Verification items for the finished model (mm, model axes). Coordinates: 2 decimals unless noted, no trailing zeros. Write each loop counter-clockwise with the first axis right and the second up, starting at its lowest first coordinate (ties: lowest second). Pieces come first, ordered by that corner, then holes. Notation, with made-up numbers: (30.5, 0.25) -> (88.5, 0.25) arc R24 ccw to (88.5, 26.25) -> close; hole circle Ø5 at (-11, 85). An arc over 180 degrees is marked (long way). Use CSV: the item, a comma, the result in double quotes.
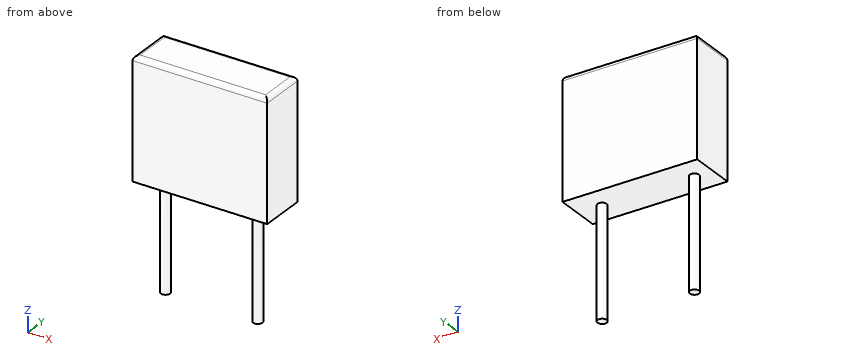
```python
from build123d import *

# Parameters (mm, degrees)
SKETCH_W     = 7.3
SKETCH_H     = 2.5
PAD_DEPTH    = 6.5
FILLET_R     = 0.25
SKETCH001_R  = 0.25
PAD001_DEPTH = 6


with BuildPart() as part:
    # Sketch → Pad (new body)
    with BuildSketch(Plane.XY):
        with Locations((0.178171, 0)):
            Rectangle(SKETCH_W, SKETCH_H)
    extrude(amount=PAD_DEPTH)

    # Fillet
    fillet_edges = [part.edges().sort_by_distance(p)[0] for p in [
        (0.178171, -1.25, 6.5),
        (0.178171, 1.25, 6.5),
        (3.828171, 0, 6.5),
        (-3.471829, 0, 6.5),
    ]]
    fillet(fillet_edges, radius=FILLET_R)

    # Sketch001 (on Face4 of Fillet) → Pad001 (join)
    with BuildSketch(Plane(origin=(0, 0, 0), x_dir=(1, 0, 0), z_dir=(0, 0, -1))):
        with Locations((2.5, 0)):
            Circle(SKETCH001_R)
        with Locations((-2.5, 0)):
            Circle(SKETCH001_R)
    extrude(amount=PAD001_DEPTH)


solid = part.part
```
1) Gauge pin test, flat ends, axial feed: pin 1 (0.8 mm diameter, centred on x = 1, y = 0, fed in from -Z); pin 2 (1 mm diameter, centred on x = 3, y = -0.5, fed in from -Z); pin 3 (3 mm diameter, centred on x = -2.5, z = -2.5, fed in from -Y); pin 4 (4 mm diameter, centred on x = -0.5, z = -4, fed in from +Y). Record the tip position at first contact, or that the pin passes through.
Return value:
pin 1,"z = 0"
pin 2,"z = -6"
pin 3,"y = -0.25"
pin 4,"y = 0.25"
2) Cross-section at B-B (x = -1.5). Record the boundary of the cut face in (y, z).
Return value:
outline,"(-1.25, 0) -> (1.25, 0) -> (1.25, 6.25) arc R0.25 ccw to (1, 6.5) -> (-1, 6.5) arc R0.25 ccw to (-1.25, 6.25) -> close"
3) Cross-section at C-C (y = 0). Record the boundary of the cut face in (x, z).
Return value:
outline,"(-3.47, 0) -> (-2.75, 0) -> (-2.75, -6) -> (-2.25, -6) -> (-2.25, 0) -> (2.25, 0) -> (2.25, -6) -> (2.75, -6) -> (2.75, 0) -> (3.83, 0) -> (3.83, 6.25) arc R0.25 ccw to (3.58, 6.5) -> (-3.22, 6.5) arc R0.25 ccw to (-3.47, 6.25) -> close"
4) Cross-section at D-D (x = -2.5). Record the boundary of the cut face in (y, z).
Return value:
outline,"(-1.25, 0) -> (-0.25, 0) -> (-0.25, -6) -> (0.25, -6) -> (0.25, 0) -> (1.25, 0) -> (1.25, 6.25) arc R0.25 ccw to (1, 6.5) -> (-1, 6.5) arc R0.25 ccw to (-1.25, 6.25) -> close"
5) Cross-section at A-A (z = -3.25). Record the boundary of the cut face in (x, y), plus the area to 3 significant figures.
Return value:
outline,"circle Ø0.5 at (-2.5, 0); circle Ø0.5 at (2.5, 0)"
area,"0.393 mm2"
6) Scan lines: L1, parallel to Z at x = -2, y = -0.95; L2, parallel to Y at x = -2.5, z = -2.5; L3, parallel to X at y = 0.1, z = -4.5. Record each from-to range of solid material in increasing order.
Return value:
L1,"0 to 6.5"
L2,"-0.25 to 0.25"
L3,"-2.73 to -2.27, 2.27 to 2.73"
